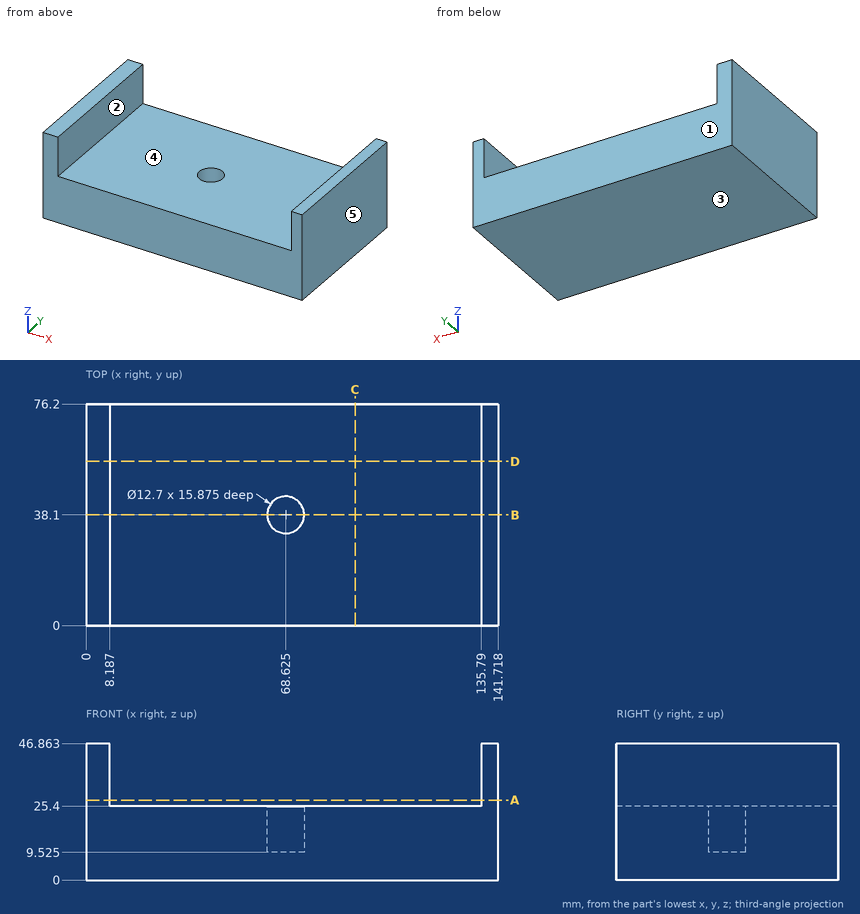
Source: three-view drawing plus pictorial views. Frame: mm from the lowest corner of the part. A direction names the side the tool comes from. Give positions to 0.01 mm unless a question says otherwise; leave off trailing zeros. Write each loop counter-clockwise with the first axis right and the second up, starting at its lowest first coordinate (ties: lowest second). Pieces come first, ordered by that corner, then holes.
(1) Access query for the marked faces 1 and 2. Directions: +Z, -Z, +X, -X, +Y, -Y. A direction counts if a zero-diameter tool reaches every point of the face in a straight line with its end or side. Return the directions, or none.
(2) Cut plane A-A, the plane z = 27.5. Return loops of the section in (x, y).
(3) First-contact query: P1, Ø14, axis at x = 71.5, y = 39.5, coming from the +Z side. Flat tip, straight axial feed; report the tip coordinate or a pass-through.
(4) Cut plane B-B, the plane y = 38.1. Return loops of the section in (x, z) (1 decimal), then the cut area to 3 significant figures.
(5) Ray query, line 1 (X direction, y = 28, z = 37); line 2 (X direction, y = 38, z = 19); line 3 (Z direction, x = 118, y = 29.5). Return the intervals inside material, ascending.
(6) Cut plane D-D, the plane y = 56.5. Return loops of the section in (x, z), then the cut area to 3 significant figures.
(7) Mould query, pull axis X, two halves, no side actions, for the marked faces 3, 4 and 5. Classes: released by +X, released by -X, zero draft, split by the parting line, or undercut.
(8) Cut plane C-C, the plane x = 92.5. Return loops of the section in (y, z).
Values follow:
1. face 1: +Z, -Z, +X, -X, +Y
1. face 2: +Z, +Y, -Y
2. outline: (0, 0) - (8.19, 0) - (8.19, 76.2) - (0, 76.2) - close; (135.79, 0) - (141.72, 0) - (141.72, 76.2) - (135.79, 76.2) - close
3. P1: stops at z = 25.4
4. outline: (0, 0) - (141.7, 0) - (141.7, 46.9) - (135.8, 46.9) - (135.8, 25.4) - (75, 25.4) - (75, 9.5) - (62.3, 9.5) - (62.3, 25.4) - (8.2, 25.4) - (8.2, 46.9) - (0, 46.9) - close
4. area: 3,700 mm2
5. line 1: x = 0 to 8.19, 135.79 to 141.72
5. line 2: x = 0 to 62.28, 74.97 to 141.72
5. line 3: z = 0 to 25.4
6. outline: (0, 0) - (141.72, 0) - (141.72, 46.86) - (135.79, 46.86) - (135.79, 25.4) - (8.19, 25.4) - (8.19, 46.86) - (0, 46.86) - close
6. area: 3,900 mm2
7. face 3: zero draft
7. face 4: undercut
7. face 5: released by +X
8. outline: (0, 0) - (76.2, 0) - (76.2, 25.4) - (0, 25.4) - close
